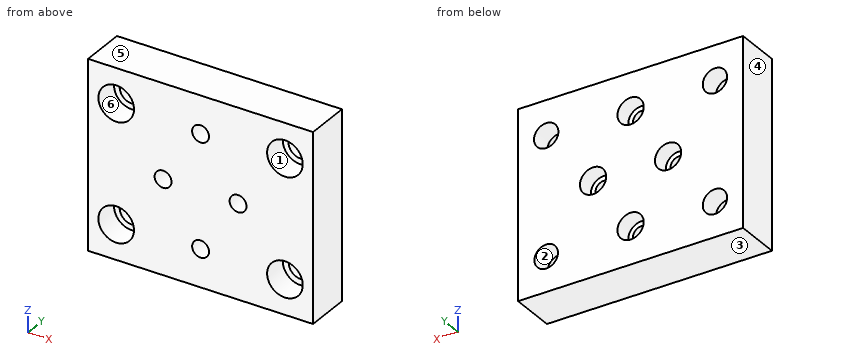
```python
from build123d import *

# Parameters (mm, degrees)
CROQUIS1_W              = 120
CROQUIS1_H              = 100
SALIENTE_EXTRUIR1_DEPTH = 24
CROQUIS2_R              = 7
CORTAR_EXTRUIR1_DEPTH   = 9
CORTAR_EXTRUIR2_REACH   = 81.53
CROQUIS3_R              = 4.5
CROQUIS4_R              = 9.5
CORTAR_EXTRUIR3_DEPTH   = 13
CROQUIS5_R              = 6.5
CROQUIS5_R_2            = 6.276895532
CORTAR_EXTRUIR4_DEPTH   = 80.177016867


with BuildPart() as part:
    # Croquis1 → Saliente-Extruir1 (new body)
    with BuildSketch(Plane(origin=(0, 0, 0), x_dir=(1, 0, 0), z_dir=(0, 1, 0))):
        Rectangle(CROQUIS1_W, CROQUIS1_H)
    extrude(amount=SALIENTE_EXTRUIR1_DEPTH)

    # Croquis2 → Cortar-Extruir1 (cut)
    with BuildSketch(Plane(origin=(0, 24, 0), x_dir=(1, 0, 0), z_dir=(0, 1, 0))):
        with Locations(Location((0, 30, 0), (0, 0, 270))):
            Circle(CROQUIS2_R)
        with Locations(Location((0, -30, 0), (0, 0, 270))):
            Circle(CROQUIS2_R)
        with Locations(Location((-20, 0, 0), (0, 0, 270))):
            Circle(CROQUIS2_R)
        with Locations(Location((20, 0, 0), (0, 0, 270))):
            Circle(CROQUIS2_R)
    extrude(amount=-CORTAR_EXTRUIR1_DEPTH, mode=Mode.SUBTRACT)

    # Croquis3 → Cortar-Extruir2 (cut, up to next)
    with BuildSketch(Plane(origin=(0, 15, 0), x_dir=(1, 0, 0), z_dir=(0, 1, 0)), mode=Mode.PRIVATE) as cortar_extruir2_sk1:
        with Locations(Location((-20, 0, 0), (0, 0, 270))):
            Circle(CROQUIS3_R)
    cortar_extruir2_tool1 = extrude(cortar_extruir2_sk1.sketch, amount=-CORTAR_EXTRUIR2_REACH, mode=Mode.PRIVATE) & part.part
    # Croquis3 → Cortar-Extruir2 (cut, up to next)
    with BuildSketch(Plane(origin=(0, 15, 0), x_dir=(1, 0, 0), z_dir=(0, 1, 0)), mode=Mode.PRIVATE) as cortar_extruir2_sk2:
        with Locations(Location((0, 30, 0), (0, 0, 270))):
            Circle(CROQUIS3_R)
    cortar_extruir2_tool2 = extrude(cortar_extruir2_sk2.sketch, amount=-CORTAR_EXTRUIR2_REACH, mode=Mode.PRIVATE) & part.part
    # Croquis3 → Cortar-Extruir2 (cut, up to next)
    with BuildSketch(Plane(origin=(0, 15, 0), x_dir=(1, 0, 0), z_dir=(0, 1, 0)), mode=Mode.PRIVATE) as cortar_extruir2_sk3:
        with Locations(Location((20, 0, 0), (0, 0, 270))):
            Circle(CROQUIS3_R)
    cortar_extruir2_tool3 = extrude(cortar_extruir2_sk3.sketch, amount=-CORTAR_EXTRUIR2_REACH, mode=Mode.PRIVATE) & part.part
    # Croquis3 → Cortar-Extruir2 (cut, up to next)
    with BuildSketch(Plane(origin=(0, 15, 0), x_dir=(1, 0, 0), z_dir=(0, 1, 0)), mode=Mode.PRIVATE) as cortar_extruir2_sk4:
        with Locations(Location((0, -30, 0), (0, 0, 270))):
            Circle(CROQUIS3_R)
    cortar_extruir2_tool4 = extrude(cortar_extruir2_sk4.sketch, amount=-CORTAR_EXTRUIR2_REACH, mode=Mode.PRIVATE) & part.part
    add(cortar_extruir2_tool1.solids().sort_by_distance((-20, 15, 0))[0], mode=Mode.SUBTRACT)
    add(cortar_extruir2_tool2.solids().sort_by_distance((0, 15, -30))[0], mode=Mode.SUBTRACT)
    add(cortar_extruir2_tool3.solids().sort_by_distance((20, 15, 0))[0], mode=Mode.SUBTRACT)
    add(cortar_extruir2_tool4.solids().sort_by_distance((0, 15, 30))[0], mode=Mode.SUBTRACT)

    # Croquis4 → Cortar-Extruir3 (cut)
    with BuildSketch(Plane.XZ):
        with Locations(Location((-45, 31.5, 0), (0, 0, 270))):
            Circle(CROQUIS4_R)
        with Locations(Location((45, 31.5, 0), (0, 0, 270))):
            Circle(CROQUIS4_R)
        with Locations(Location((45, -31.5, 0), (0, 0, 270))):
            Circle(CROQUIS4_R)
        with Locations(Location((-45, -31.5, 0), (0, 0, 270))):
            Circle(CROQUIS4_R)
    extrude(amount=-CORTAR_EXTRUIR3_DEPTH, mode=Mode.SUBTRACT)

    # Croquis5 → Cortar-Extruir4 (cut, through all)
    with BuildSketch(Plane.XZ.offset(-13)):
        with Locations(Location((-45, 31.5, 0), (0, 0, 270))):
            Circle(CROQUIS5_R)
        with Locations(Location((45, 31.5, 0), (0, 0, 270))):
            Circle(CROQUIS5_R)
        with Locations(Location((-45, -31.5, 0), (0, 0, 270))):
            Circle(CROQUIS5_R)
        with Locations(Location((45, -31.5, 0), (0, 0, 270))):
            Circle(CROQUIS5_R_2)
    extrude(amount=-CORTAR_EXTRUIR4_DEPTH, mode=Mode.SUBTRACT)


solid = part.part
```
Verification items for the finished model (mm, model axes). Face numbers are marked on the shaded views. A direction names the side the tool comes from. Give positions to 0.01 mm unless a question says otherwise; leave off trailing zeros. Loops run counter-clockwise (first coordinate to the right, second up) from the corner with the lowest first, then second, coordinate; pieces in that order, holes last. Notation, with made-up numbers: M 50,54.5 L 81,54.5 A15 ccw 81,74.5 Z; hole C 5.25,-12.75 d4. An arc over 180 degrees is marked long. Return JSON: item names as keys, results as strings.
1) Gauge pin test, flat ends, axial feed: P1, Ø11.5, axis at x = -20, z = 0, coming from the +Y side; P2, Ø17, axis at x = 45, z = 31.5, coming from the -Y side. Record the tip position at first contact, or that the pin passes through.
Findings:
{"P1": "stops at y = 15", "P2": "stops at y = 13"}
2) Material ranges on L1, parallel to X at y = 17.75, z = 0; L2, parallel to X at y = 5, z = 0; L3, parallel to X at y = 5.75, z = -31.5, recorded low to high. Write a range as [from, to].
Findings:
{"L1": "x = [-60, -27], [-13, 13], [27, 60]", "L2": "x = [-60, -24.5], [-15.5, 15.5], [24.5, 60]", "L3": "x = [-60, -54.5], [-35.5, -4.24], [4.24, 35.5], [54.5, 60]"}
3) Section check C-C, the plane y = 19.75. Count the separate pieces of the cut face and the enclosed holes in it, and give its area (3 significant figures).
Findings:
{"separate pieces": "1", "enclosed holes": "8", "area": "10,900 mm2"}
4) Section check D-D, the plane x = 20. Enter the section's corners in (y, z), and give its area (3 significant figures).
Findings:
{"outline": "M 0,-50 L 24,-50 L 24,-7 L 15,-7 L 15,-4.5 L 0,-4.5 Z; M 0,4.5 L 15,4.5 L 15,7 L 24,7 L 24,50 L 0,50 Z", "area": "2,140 mm2"}
5) Tool access check on the marked faces 5 and 6. Record the directions out of +Z, -Z, +X, -X, +Y, -Y that give a thin tool (end or side, any length) a straight path to the whole face; none if there is none.
Findings:
{"face 5": "+Z, +X, -X, +Y, -Y", "face 6": "-Y"}
6) Section check A-A, the plane z = 0. Enter the section's corners in (x, y).
Findings:
{"outline": "M -60,0 L -24.5,0 L -24.5,15 L -27,15 L -27,24 L -60,24 Z; M -15.5,0 L 15.5,0 L 15.5,15 L 13,15 L 13,24 L -13,24 L -13,15 L -15.5,15 Z; M 24.5,0 L 60,0 L 60,24 L 27,24 L 27,15 L 24.5,15 Z"}
7) Mould release check, pull along X, two halves, no side actions. Record for the marked faces 1, 2, 3 and 4: released by +X, released by -X, zero draft, split by the parting line, or undercut.
Findings:
{"face 1": "undercut", "face 2": "undercut", "face 3": "zero draft", "face 4": "released by -X"}
8) Section check B-B, the plane x = 45. Enter the section's corners in (y, z).
Findings:
{"outline": "M 0,-50 L 24,-50 L 24,-37.78 L 13,-37.78 L 13,-41 L 0,-41 Z; M 0,-22 L 13,-22 L 13,-25.22 L 24,-25.22 L 24,25 L 13,25 L 13,22 L 0,22 Z; M 0,41 L 13,41 L 13,38 L 24,38 L 24,50 L 0,50 Z"}
